```python
from build123d import *

# Parameters (mm, degrees)
F3_ANGLE_BACK  = 22.5
F3_ANGLE       = 45
F5_START       = 4.7625
F5_DEPTH       = 73.661
F7_DEPTH       = 78.4235
F8_COUNT       = 3
F9_R           = 1.27
F10_DEPTH      = 50.8733057387
F10_DEPTH_BACK = 76.59454776


with BuildPart() as f1:
    # F0 (on Front) → F1 (revolve)
    with BuildSketch(Plane.XZ):
        Polygon((13.2207, 50.8), (13.2207, 78.4225), (8.4582, 78.4225), (8.4582, 55.5625), (4.191, 55.5625), (4.191, 50.8), align=None)
    revolve(axis=Axis((0, 0, 76.2090291828), (0, 0, 1)))

    # F2 (on Front) → F3 (revolve)
    with BuildSketch(Plane.XZ, mode=Mode.PRIVATE) as f3_sk:
        Polygon((50.40645224, 4.7625), (13.2207, 66.3656993785), (13.2207, 57.15), (44.84354776, 4.7625), (38.49354776, 4.7625), (38.49354776, 0), (76.59354776, 0), (76.59354776, 4.7625), align=None)
    revolve(f3_sk.sketch.rotate(Axis((0, 0, 76.2090291828), (0, 0, 1)), -F3_ANGLE_BACK), axis=Axis((0, 0, 76.2090291828), (0, 0, 1)), revolution_arc=F3_ANGLE)

    # F4 (on Top) → F5 (cut)
    with BuildSketch(Plane.XY.offset(F5_START)):
        Polygon((12.2143341355, 33.2312490207), (12.2143341355, 5.0593428543), (63.5, 5.0593428543), (63.5, -5.0593428543), (12.2143341355, -5.0593428543), (12.2143341355, -33.2312490207), (78.2526575172, -33.2312490207), (78.2526575172, 33.2312490207), align=None)
    extrude(amount=F5_DEPTH, mode=Mode.SUBTRACT)

    # F6 (on Top) → F7 (cut, through all)
    with BuildSketch(Plane.XY):
        Polygon((50.1519040247, 31.7581439537), (50.1519040247, 20.7735988259), (87.7114310861, 12.7), (87.7114310861, -12.7), (50.1519040247, -20.7735988259), (50.1519040247, -36.5923251011), (108.705951746, -36.5923251011), (108.705951746, 31.7581439537), align=None)
    extrude(amount=F7_DEPTH, mode=Mode.SUBTRACT)

    # F8: F1 ×3 about axis
    f8_axis = Axis((0, 0, 76.2090291828), (0, 0, 1))


with BuildPart() as f1_1:
    add(f1.part)
    for i in range(1, F8_COUNT):
        add(f1.part.rotate(f8_axis, i * 360 / F8_COUNT))

    # F9 (on Right) → F10 (cut, two sides)
    with BuildSketch(Plane.YZ) as f10_sk:
        with Locations((-7.9375, 71.4375)):
            Circle(F9_R)
        with Locations((7.9375, 71.4375)):
            Circle(F9_R)
    extrude(amount=-F10_DEPTH, mode=Mode.SUBTRACT)
    extrude(f10_sk.sketch, amount=F10_DEPTH_BACK, mode=Mode.SUBTRACT)


solid = f1_1.part
```
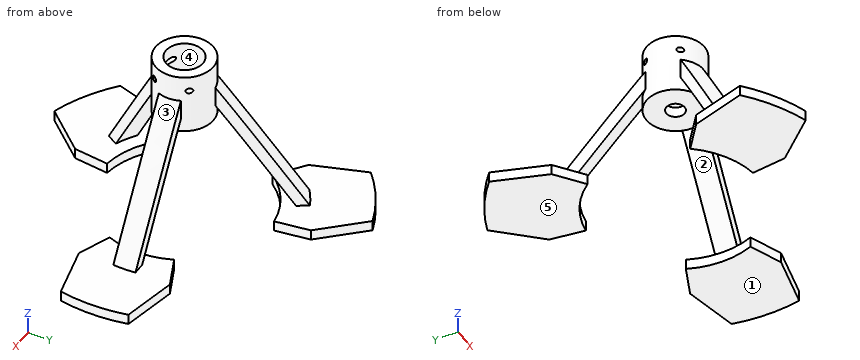
The model under review builds one solid part; all positions refer to its coordinate system, in mm. Face numbers are marked on the shaded views. A direction names the side the tool comes from. Round coordinates to 2 decimals unless told otherwise and drop trailing zeros. Order: outer loops, then holes, each group sorted by start corner. A loop starts at its lowest first (then second) coordinate and runs counter-clockwise, first axis right, second up. Notation, with made-up numbers: (-37, 58) -> (-15, 58) arc R9 cw to (-15, 71) -> close; hole circle Ø8 at (12.5, -20.5). An arc over 180 degrees is marked (long way). Use a Markdown table: item, result.
Q1. We need section B-B on x = -34. Write out the cut boundary in (y, z).
Values:
| item | result |
|---|---|
| outline | (-68.63, 0) -> (-26.09, 0) -> (-26.09, 4.76) -> (-68.63, 4.76) -> close; (26.09, 0) -> (68.63, 0) -> (68.63, 4.76) -> (26.09, 4.76) -> close |
Q2. Clearance check with flat-ended pins moving along their axes: P1, Ø5, axis at x = 0, y = 0, coming from the -Z side; P2, Ø10, axis at x = 14.5, z = 50, coming from the +Y side; P3, Ø23, axis at x = -36, y = 60, coming from the +Z side; P4, Ø19, axis at x = 28, z = 20.5, coming from the -Y side. State where each tip first meets the part, or that it passes through.
Values:
| item | result |
|---|---|
| P1 | passes through |
| P2 | stops at y = 9.13 |
| P3 | stops at z = 4.76 |
| P4 | stops at y = -5.06 |
Q3. We need section C-C on z = 29. Write out the cut boundary in (x, y), then the cut area to 3 significant figures.
Values:
| item | result |
|---|---|
| outline | (-22.09, -28.14) arc R35.78 ccw to (-13.33, -33.2) -> (-10.51, -28.33) arc R30.21 cw to (-19.27, -23.27) -> close; (-22.09, 28.14) -> (-19.27, 23.27) arc R30.21 cw to (-10.51, 28.33) -> (-13.33, 33.2) arc R35.78 ccw to start; (29.79, -5.06) -> (35.42, -5.06) arc R35.78 ccw to (35.42, 5.06) -> (29.79, 5.06) arc R30.21 cw to start |
| area | 170 mm^2 |
Q4. We need section D-D on z = 48. Write out the cut boundary in (x, y).
Values:
| item | result |
|---|---|
| outline | (-16.27, -18.06) arc R24.31 ccw to (-7.51, -23.12) -> (-4.64, -18.16) arc R18.74 cw to (-13.41, -13.1) -> close; (-16.27, 18.06) -> (-13.41, 13.1) arc R18.74 cw to (-4.64, 18.16) -> (-7.51, 23.12) arc R24.31 ccw to start; (18.05, -5.06) -> (23.77, -5.06) arc R24.31 ccw to (23.77, 5.06) -> (18.05, 5.06) arc R18.74 cw to start |
Q5. Tool access review of the marked faces 4 and 5: name each direction out of +Z, -Z, +X, -X, +Y, -Y from which nothing blocks a thin tool from reaching the whole face with its end or side.
Values:
| item | result |
|---|---|
| face 4 | +Z |
| face 5 | -Z, +X, -X, +Y, -Y |
Q6. We need section A-A on y = 0. Write out the cut boundary in (x, z), then the cut area to 3 significant figures.
Values:
| item | result |
|---|---|
| outline | (-13.22, 50.8) -> (-4.19, 50.8) -> (-4.19, 55.56) -> (-8.46, 55.56) -> (-8.46, 78.42) -> (-13.22, 78.42) -> close; (4.19, 50.8) -> (13.22, 50.8) -> (13.22, 57.15) -> (44.84, 4.76) -> (38.49, 4.76) -> (38.49, 0) -> (76.59, 0) -> (76.59, 4.76) -> (50.41, 4.76) -> (13.22, 66.37) -> (13.22, 78.42) -> (8.46, 78.42) -> (8.46, 55.56) -> (4.19, 55.56) -> close |
| area | 802 mm^2 |
Q7. For line 1 (X direction, y = 0, z = 70); line 2 (Y direction, x = 0, z = 53.3), list the stretches that pass through material, from the lowest coordinate up.
Values:
| item | result |
|---|---|
| line 1 | x = -13.22 to -8.46, 8.46 to 13.22 |
| line 2 | y = -13.22 to -4.19, 4.19 to 13.22 |
Q8. Mouldability with a two-part tool opening along Y and no side actions: class the marked faces 1, 2 and 3 as +Y half, -Y half, draft (parallel to the pull), parting line (faces both ways), or undercut.
Values:
| item | result |
|---|---|
| face 1 | draft |
| face 2 | undercut |
| face 3 | parting line |
